from build123d import *

# Parameters (mm, degrees)
F0_R     = 25
F0_R_2   = 2.5
F1_DEPTH = 60
F2_DEPTH = 60
F3_SIZE  = 3


with BuildPart() as f1:
    # F0 (on Top) → F1 (new body)
    with BuildSketch(Plane.XY):
        Circle(F0_R)
        Circle(F0_R_2, mode=Mode.SUBTRACT)
        Circle(F0_R_2)
    extrude(amount=F1_DEPTH)

    # F0 (on Top) → F2 (cut)
    with BuildSketch(Plane.XY):
        Circle(F0_R_2)
    extrude(amount=F2_DEPTH, mode=Mode.SUBTRACT)

    # F3
    f3_edges = [f1.edges().sort_by_distance(p)[0] for p in [
        (-25, 0, 60),
        (-25, 0, 0),
    ]]
    chamfer(f3_edges, length=F3_SIZE)


solid = f1.part
Here's how the part is built. I have some questions about the finished solid (model axes, mm). Coordinates: 2 decimals unless noted, no trailing zeros. Write each loop counter-clockwise with the first axis right and the second up, starting at its lowest first coordinate (ties: lowest second). Pieces come first, ordered by that corner, then holes.
1) If we section it at A-A (x = 0): List the corners of the cut face in (y, z) for me.
Filled in:
outline: (-25, 3) - (-22, 0) - (-2.5, 0) - (-2.5, 60) - (-22, 60) - (-25, 57) - close; (2.5, 0) - (22, 0) - (25, 3) - (25, 57) - (22, 60) - (2.5, 60) - close
2) I'm going to push flat-ended pins straight in: pin 1 (1.5 mm diameter, centred on x = -17.5, z = 36, fed in from +Y); pin 2 (12 mm diameter, centred on x = 1.5, z = 21.5, fed in from +Y); pin 3 (10 mm diameter, centred on x = 12, z = 10, fed in from -Y). Where does each tip first touch, or does it pass through?
Filled in:
pin 1: stops at y = 18.56
pin 2: stops at y = 25
pin 3: stops at y = -24
3) If I drill on line 1 (Y direction, x = 0, z = 21); line 2 (Y direction, x = -1.5, z = 42); line 3 (X direction, y = 13.5, z = 40), over which ranges is the centre line in solid material (lowest first)?
Filled in:
line 1: y = -25 to -2.5, 2.5 to 25
line 2: y = -24.95 to -2, 2 to 24.95
line 3: x = -21.04 to 21.04
4) If we section it at C-C (z = 23): List the corners of the cut face in (x, y) for me.
Filled in:
outline: circle Ø50 at (0, 0); hole circle Ø5 at (0, 0)
